Read the model definition and answer for the solid it produces. Units are mm, in the model's axes. A direction names the side the tool comes from. Coordinates: 2 decimals unless noted, no trailing zeros. Loops run counter-clockwise (first coordinate to the right, second up) from the corner with the lowest first, then second, coordinate; pieces in that order, holes last. Notation, with made-up numbers: M -10,27 L 21,27 A20 ccw 21,36 Z; hole C 73,34 d3. An arc over 180 degrees is marked long. Put each result on its own line as item: value.
from build123d import *

# Parameters (mm, degrees)
F0_R     = 2.25
F1_DEPTH = 7
F0_W     = 7
F0_H     = 6
F2_DEPTH = 11
F4_D     = 2.8
F4_DEPTH = 11
F4_TIP   = 0.8412048666


with BuildPart() as f1:
    # F0 (on Top) → F1 (new body)
    with BuildSketch(Plane.XY):
        Polygon((-22.5828918815, 30.6862212941), (-42.5828918815, 30.6862212941), (-42.5828918815, 18.1862212941), (-35.5828918815, 18.1862212941), (-35.5828918815, 12.1862212941), (-42.5828918815, 12.1862212941), (-42.5828918815, 5.1862212941), (-22.5828918815, 5.1862212941), align=None)
        with Locations((-27.5828918815, 15.1862212941)):
            Circle(F0_R, mode=Mode.SUBTRACT)
    extrude(amount=F1_DEPTH)

    # F0 (on Top) → F2 (join)
    with BuildSketch(Plane.XY):
        with Locations((-39.0828918815, 15.1862212941)):
            Rectangle(F0_W, F0_H)
    extrude(amount=F2_DEPTH)

    # F4
    with Locations(Plane(origin=(0, 30.6862212941, 0), x_dir=(-1, 0, 0), z_dir=(0, 1, 0))):
        with Locations((32.5828918815, 3.5)):
            Hole(F4_D / 2, depth=F4_DEPTH)
            with Locations((0, 0, -(F4_DEPTH + F4_TIP / 2))):  # 118° drill point
                Cone(0, F4_D / 2, F4_TIP, mode=Mode.SUBTRACT)


solid = f1.part
1) Find section A-A, the plane y = 16.5. Write down the section's boundary in (x, z).
Answer list:
outline: M -42.58,0 L -29.41,0 L -29.41,7 L -35.58,7 L -35.58,11 L -42.58,11 Z; M -25.76,0 L -22.58,0 L -22.58,7 L -25.76,7 Z
2) Given pin 1 Ø4 at (x, y) = (-33, 24) entering from +Z; pin 2 Ø3 at (y, z) = (14, 9) entering from +X; pin 3 Ø2.5 at (x, y) = (-27.58, 15.19) entering from -Z; pin 4 Ø3 at (x, z) = (-37.5, 10) entering from -Y, each flat-ended and moving along its own axis, determine where each tip first touches the part or whether it passes through.
Answer list:
pin 1: stops at z = 7
pin 2: stops at x = -35.58
pin 3: passes through
pin 4: stops at y = 12.19
3) Straight lines are drawn through the part: line 1 (X direction, y = 27, z = 3.5); line 2 (Z direction, x = -38.75, y = 22); line 3 (Y direction, x = -37, z = 8). For each, find the intervals that lie inside material, in ascending order. Write a range as [from, to].
Answer list:
line 1: x = [-42.58, -33.98], [-31.18, -22.58]
line 2: z = [0, 7]
line 3: y = [12.19, 18.19]
4) Which of the six approach directions +Z, -Z, +X, -X, +Y, -Y give full straight-line access (tool end or side, diameter ignored) to faces 1 (the flat face through (-35.583, 15, 9)), 2 (the flat face through (-39, 18.186, 9)), 3 (the flat face through (-39, 12.186, 9))?
Answer list:
face 1: +Z, +X, +Y, -Y
face 2: +Z, +X, -X, +Y
face 3: +Z, +X, -X, -Y
5) Find section D-D, the plane y = 20. Write down the section's boundary in (x, z), plus the area to 3 significant figures.
Answer list:
outline: M -42.58,0 L -22.58,0 L -22.58,7 L -42.58,7 Z; hole C -32.58,3.5 d2.8
area: 134 mm^2
6) Find section C-C, the plane z = 1. Write down the section's boundary in (x, y), plus the area to 3 significant figures.
Answer list:
outline: M -42.58,5.19 L -22.58,5.19 L -22.58,30.69 L -42.58,30.69 Z; hole C -27.58,15.19 d4.5
area: 494 mm^2
7) Find section B-B, the plane x = -41. Write down the section's boundary in (y, z), plus the area to 4 significant figures.
Answer list:
outline: M 5.19,0 L 30.69,0 L 30.69,7 L 18.19,7 L 18.19,11 L 12.19,11 L 12.19,7 L 5.19,7 Z
area: 202.5 mm^2
8) Determine the mould class of faces 4 (the flat face through (-39, 15, 11)), 5 (the cylindrical face through (-28.07, 12.99, 3.45)), 6 (the cylindrical face through (-33.98, 25.11, 3.56)) for opening direction Z: released by +Z, released by -Z, zero draft, split by the parting line, or undercut.
Answer list:
face 4: released by +Z
face 5: zero draft
face 6: undercut
